Study the drawing (mm; zero at the part's minimum x, y, z) and answer. A direction names the side the tool comes from. Round coordinates to 2 decimals unless told otherwise and drop trailing zeros. Write each loop counter-clockwise with the first axis right and the second up, starting at its lowest first coordinate (ties: lowest second). Pieces come first, ordered by that corner, then holes. Notation, with made-up numbers: (65.25, -32) - (93.25, -32) arc R13 cw to (93.25, -23) - close; hole circle Ø9 at (-16, 18.5). An arc over 180 degrees is marked (long way). Return JSON: item names as keys, results as strings. Group by question number.
(1) Which of the six approach directions +Z, -Z, +X, -X, +Y, -Y give full straight-line access (tool end or side, diameter ignored) to the marked faces 1, 2 and 3?
(2) Section A-A, the plane z = 8 is taken. Write down the section's boundary in (x, y).
(3) Section C-C, the plane x = 55.5 is taken. Write down the section's boundary in (y, z), then the cut area to 3 significant figures.
(4) Section B-B, the plane y = 69 is taken. Write down the section's boundary in (x, z), then the cut area to 3 significant figures.
(5) Each of these flat-tipped pins is pushed along its axis until it touches: pin 1 (6 mm diameter, centred on x = 18.5, z = 9, fed in from +Y); pin 2 (3.5 mm diameter, centred on x = 7.5, y = 30.5, fed in from -Z); pin 3 (3 mm diameter, centred on x = 75, y = 83.5, fed in from +Z); pin 4 (1 mm diameter, centred on y = 38, z = 3, fed in from +X). Where does it stop, or does it pass through?
(6) Determine the mould class of the marked faces 4 and 5 for opening direction X: +X half, -X half, draft (parallel to the pull), parting line (faces both ways), or undercut.
(7) Find the intervals of material crossed by line 1 along X through (y, z) = (37, 8.75); line 2 along Z through (x, y) = (82, 10); line 3 along X through (y, z) = (12, 2), in increasing order. Write a range as [from, to].
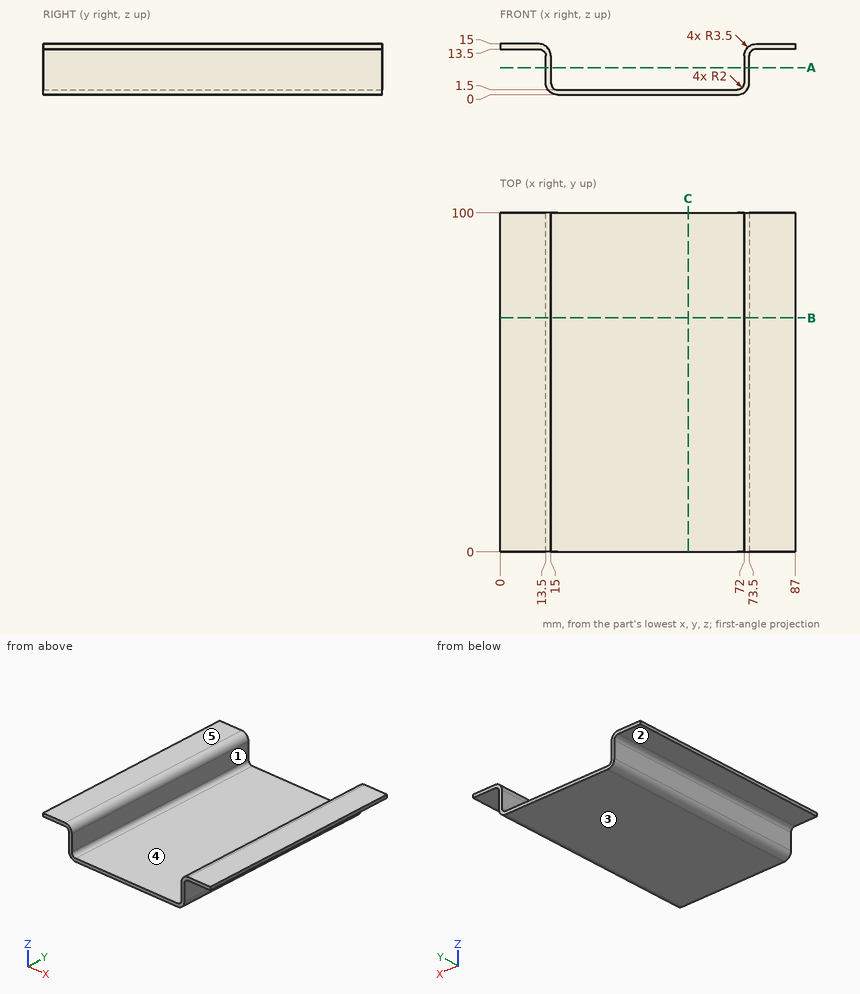
Working result:
{
 "1": {"face 1": "+Z, +Y, -Y", "face 2": "-Z, -X, +Y, -Y", "face 3": "-Z, +X, -X, +Y, -Y"},
 "2": {"outline": "(13.5, 0) - (15, 0) - (15, 100) - (13.5, 100) - close; (72, 0) - (73.5, 0) - (73.5, 100) - (72, 100) - close"},
 "3": {"outline": "(0, 0) - (100, 0) - (100, 1.5) - (0, 1.5) - close", "area": "150 mm^2"},
 "4": {"outline": "(0, 13.5) - (11.5, 13.5) arc R2 cw to (13.5, 11.5) - (13.5, 3.5) arc R3.5 ccw to (17, 0) - (70, 0) arc R3.5 ccw to (73.5, 3.5) - (73.5, 11.5) arc R2 cw to (75.5, 13.5) - (87, 13.5) - (87, 15) - (75.5, 15) arc R3.5 ccw to (72, 11.5) - (72, 3.5) arc R2 cw to (70, 1.5) - (17, 1.5) arc R2 cw to (15, 3.5) - (15, 11.5) arc R3.5 ccw to (11.5, 15) - (0, 15) - close", "area": "164 mm^2"},
 "5": {"pin 1": "passes through", "pin 2": "stops at z = 13.5", "pin 3": "stops at z = 15", "pin 4": "stops at x = 73.5"},
 "6": {"face 4": "undercut", "face 5": "draft"},
 "7": {"line 1": "x = [13.5, 15], [72, 73.5]", "line 2": "z = [13.5, 15]", "line 3": "x = [13.84, 15.68], [71.32, 73.16]"}
}
